from build123d import *

# Parameters (mm, degrees)
SKETCH_1_W          = 9
SKETCH_1_H          = 15
EXTRUDE_1_DEPTH     = 90
SKETCH_2_R          = 2.1
CUT_EXTRUDE_1_DEPTH = 6
SKETCH_3_W          = 5
SKETCH_3_H          = 2.25
EXTRUDE_2_DEPTH     = 3
CHAMFER_1_SIZE      = 0.75
EXTRUDE_3_DEPTH     = 9
SKETCH_4_R          = 2.1
CUT_EXTRUDE_2_DEPTH = 6


with BuildPart() as part:
    # Эскиз1 → Бобышка-Вытянуть1 (new body)
    with BuildSketch(Plane.XY):
        Rectangle(SKETCH_1_W, SKETCH_1_H)
        Polygon((-4.5, 12.25), (-4.5, 7.5), (-0.5, 7.5), (-0.5, 9.75), (4.5, 9.75), (4.5, 12.25), align=None)
    extrude(amount=EXTRUDE_1_DEPTH)

    # Эскиз2 → Вырез-Вытянуть1 (cut)
    with BuildSketch(Plane.XZ.offset(7.5)):
        with Locations(Location((0, 22.5, 0), (0, 0, 270))):
            Circle(SKETCH_2_R)
        with Locations(Location((0, 67.5, 0), (0, 0, 270))):
            Circle(SKETCH_2_R)
        with Locations(Location((0, 45, 0), (0, 0, 270))):
            Circle(SKETCH_2_R)
    extrude(amount=-CUT_EXTRUDE_1_DEPTH, mode=Mode.SUBTRACT)

    # Эскиз3 → Бобышка-Вытянуть2 (add)
    with BuildSketch(Plane(origin=(0, 0, 90), x_dir=(-1, 0, 0), z_dir=(0, 0, -1))):
        with Locations((-2, 8.625)):
            Rectangle(SKETCH_3_W, SKETCH_3_H)
    extrude(amount=EXTRUDE_2_DEPTH)

    # Фаска1
    chamfer_1_edges = [part.edges().sort_by_distance(p)[0] for p in [
        (4.5, 9.75, 43.5),
        (4.5, 7.5, 43.5),
    ]]
    chamfer(chamfer_1_edges, length=CHAMFER_1_SIZE)

    # Эскиз5 → Бобышка-Вытянуть3 (add)
    with BuildSketch(Plane.ZY.offset(4.5)):
        Polygon((0, 12.25), (0, 37.25), (4.84785343, 37.25), (29.84785343, 12.25), align=None)
    extrude(amount=-EXTRUDE_3_DEPTH)

    # Эскиз4 → Вырез-Вытянуть2 (cut)
    with BuildSketch(Plane(origin=(0, 0, 0), x_dir=(-1, 0, 0), z_dir=(0, 0, -1))):
        with Locations((0, 2.5)):
            Circle(SKETCH_4_R)
        with Locations((0, 27.25)):
            Circle(SKETCH_4_R)
    extrude(amount=-CUT_EXTRUDE_2_DEPTH, mode=Mode.SUBTRACT)


with BuildPart() as body_2:
    # Зеркальное отражение1: mirrored copy
    add(part.part.mirror(Plane(origin=(-4.5, 0, 90), x_dir=(0, 0, 1), z_dir=(-1, 0, 0))))


solid = body_2.part
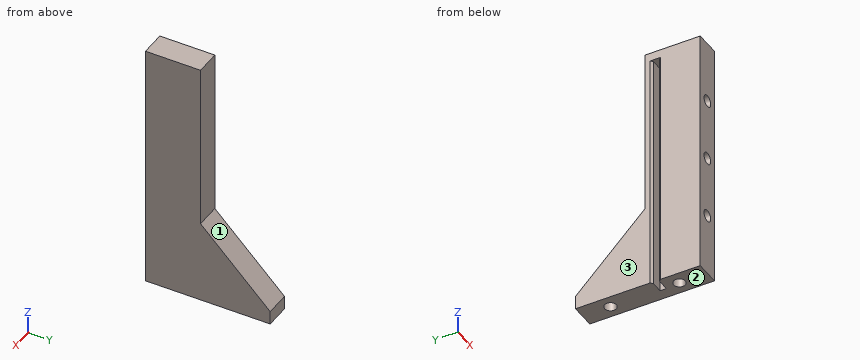
Verification items for the finished model (mm, model axes). Face numbers are marked on the shaded views. Coordinates: 2 decimals unless noted, no trailing zeros. Order: outer loops, then holes, each group sorted by start corner. A loop starts at its lowest first (then second) coordinate and runs counter-clockwise, first axis right, second up. Notation, with made-up numbers: (10, 5) -> (60, 5) arc R22 ccw to (60, 32) -> close; hole circle Ø8 at (41.5, 71.5). An arc over 180 degrees is marked (long way). Put each result on its own line as item: value. Start each with the question number.
1. Mould release check, pull along Z, two halves, no side actions. Record for the marked faces 1, 2 and 3: released by +Z, released by -Z, zero draft, split by the parting line, or undercut.
2. Cross-section at C-C, the plane y = 2.5. Record the boundary of the cut face in (x, z), then the cut area to 3 significant figures.
3. Go/stop test with flat-tipped pins: pin 1 Ø3.5 at (x, z) = (-9, 45) entering from -Y; pin 2 Ø2.5 at (y, z) = (8.5, 54.5) entering from -X; pin 3 Ø3.5 at (x, y) = (-9, 27) entering from -Z. Record where each tip stops, or that it passes through.
4. Cross-section at A-A, the plane y = -2.5. Record the boundary of the cut face in (x, z).
5. Cross-section at B-B, the plane z = 39. Record the boundary of the cut face in (x, y).
6. Material ranges on L1, parallel to Z at x = -9, y = -3.95; L2, parallel to Z at x = -8.25, y = -4.5; L3, parallel to X at y = -5.2, z = 45, recorded low to high. Write a range as [from, to].
7. Cross-section at D-D, the plane z = 22.5. Record the boundary of the cut face in (x, y).
Computed:
1. face 1: released by +Z
1. face 2: released by -Z
1. face 3: zero draft
2. outline: (-13.5, 0) -> (-11.1, 0) -> (-11.1, 6) -> (-6.9, 6) -> (-6.9, 0) -> (-4.5, 0) -> (-4.5, 90) -> (-13.5, 90) -> close
2. area: 785 mm2
3. pin 1: y = -1.5
3. pin 2: x = -13
3. pin 3: z = 6
4. outline: (-13.5, 0) -> (-4.5, 0) -> (-4.5, 90) -> (-13.5, 90) -> close; hole circle Ø4.2 at (-9, 22.5); hole circle Ø4.2 at (-9, 45); hole circle Ø4.2 at (-9, 67.5)
5. outline: (-13.5, -7.5) -> (-4.5, -7.5) -> (-4.5, 12.25) -> (-13.5, 12.25) -> (-13.5, 10.5) -> (-12.75, 9.75) -> (-8.5, 9.75) -> (-8.5, 7.5) -> (-12.75, 7.5) -> (-13.5, 6.75) -> close
6. L1: [0, 20.4], [24.6, 42.9], [47.1, 65.4], [69.6, 90]
6. L2: [0, 20.54], [24.46, 43.04], [46.96, 65.54], [69.46, 90]
6. L3: [-13.5, -11.1], [-6.9, -4.5]
7. outline: (-13.5, -7.5) -> (-11.1, -7.5) -> (-11.1, -1.5) -> (-6.9, -1.5) -> (-6.9, -7.5) -> (-4.5, -7.5) -> (-4.5, 19.6) -> (-13.5, 19.6) -> (-13.5, 10.5) -> (-12.75, 9.75) -> (-8.5, 9.75) -> (-8.5, 7.5) -> (-12.75, 7.5) -> (-13.5, 6.75) -> close
